from build123d import *

# Parameters (mm, degrees)
F2_W          = 2.032
F2_H          = 3.556
F2_W_2        = 3.556
F2_H_2        = 2.032
F3_DEPTH      = 25.4
F3_DEPTH_BACK = 4.3434


# Not quite as in the source:
# - a feature names something its author has since deleted; it is built from what else it names


with BuildPart() as f1:
    # F0 (on Front) → F1 (revolve)
    with BuildSketch(Plane.XZ):
        with BuildLine():
            ThreePointArc((8.3732076521, 7.5855466623), (7.9877835669, 8.7130510839), (6.9264967271, 9.2547965866))
            Line((6.9264967271, 9.2547965866), (-0.5167923479, 9.906))
            Line((-0.5167923479, 9.906), (-4.3267923479, 9.906))
            Line((-4.3267923479, 9.906), (-4.3267923479, 8.73125))
            Line((-4.3267923479, 8.73125), (-7.5017923479, 8.73125))
            Line((-7.5017923479, 8.73125), (-7.5017923479, 7.5438))
            Line((-7.5017923479, 7.5438), (-13.4549173479, 7.5438))
            ThreePointArc((-13.4549173479, 7.5438), (-13.7355503517, 7.4275580038), (-13.8517923479, 7.146925))
            Line((-13.8517923479, 7.146925), (-13.8517923479, 6.5024))
            Line((-13.8517923479, 6.5024), (8.3732076521, 6.5024))
            Line((8.3732076521, 6.5024), (8.3732076521, 7.5855466623))
        make_face()
    revolve(axis=Axis((-0.2325048039, 0, 0), (1, 0, 0)))

    # F2 (on Right) → F3 (cut, two sides)
    with BuildSketch(Plane.YZ) as f3_sk:
        with Locations((0, -8.1534)):
            Rectangle(F2_W, F2_H)
        with Locations((0, 8.1534)):
            Rectangle(F2_W, F2_H)
        with Locations((-8.1534, 0)):
            Rectangle(F2_W_2, F2_H_2)
        with Locations((8.1534, 0)):
            Rectangle(F2_W_2, F2_H_2)
    extrude(amount=F3_DEPTH, mode=Mode.SUBTRACT)
    extrude(f3_sk.sketch, amount=-F3_DEPTH_BACK, mode=Mode.SUBTRACT)


solid = f1.part
The model under review builds one solid part; all positions refer to its coordinate system, in mm. A direction names the side the tool comes from. Coordinates: 2 decimals unless noted, no trailing zeros. Write each loop counter-clockwise with the first axis right and the second up, starting at its lowest first coordinate (ties: lowest second). Pieces come first, ordered by that corner, then holes. Notation, with made-up numbers: M 54.25,1 L 76.25,1 A21 cw 76.25,29 Z; hole C -29.75,19.25 d3. An arc over 180 degrees is marked long. Put each result on its own line as item: value.
1) Add section D-D on x = -10. Give the boundary of the cut face in (y, z), then the cut area to 3 significant figures.
Computed:
outline: C 0,0 d15.09; hole C 0,0 d13
area: 46.0 mm2
2) For faces 1 (the flat face through (2, 1.016, 8)), 2 (the flat face through (2, -8, 1.016)), 3 (the flat face through (-7.502, 4, -7)), list the 3-axis set-ups (+Z, -Z, +X, -X, +Y, -Y) from which the entire face can be reached by the end or side of a thin tool; tool diameter is ignored.
Computed:
face 1: +Z, -Z, +X
face 2: +X, +Y, -Y
face 3: -X
3) Add section B-B on x = -2.75. Give the boundary of the cut face in (y, z), then the cut area to 3 significant figures.
Computed:
outline: M -9.85,-1.02 A9.91 ccw -1.02,-9.85 L -1.02,-6.42 A6.5 cw -6.42,-1.02 Z; M -9.85,1.02 L -6.42,1.02 A6.5 cw -1.02,6.42 L -1.02,9.85 A9.91 ccw Z; M 1.02,-9.85 A9.91 ccw 9.85,-1.02 L 6.42,-1.02 A6.5 cw 1.02,-6.42 Z; M 1.02,6.42 A6.5 cw 6.42,1.02 L 9.85,1.02 A9.91 ccw 1.02,9.85 Z
area: 148 mm2
4) Clearance check with flat-ended pins moving along their axes: pin 1 Ø4 at (x, z) = (1, -9) entering from -Y; pin 2 Ø1 at (y, z) = (0, -7.5) entering from +X; pin 3 Ø4 at (x, z) = (2, -8.5) entering from +Y; pin 4 Ø4 at (y, z) = (0, 3.5) entering from +X. State where each tip first meets the part, or that it passes through.
Computed:
pin 1: stops at y = -6.84
pin 2: stops at x = -4.34
pin 3: stops at y = 7.2
pin 4: passes through
5) Draft analysis for pull direction Y (two halves, no side actions). For faces 4 (the flat face through (-4.343, 0, -8)), 5 (the cylindrical face through (-2.45, 6.94, -7.07)), 6 (the flat face through (8.373, -5, 5)), state which applies: released by +Y, released by -Y, zero draft, split by the parting line, or undercut.
Computed:
face 4: undercut
face 5: released by +Y
face 6: zero draft
6) Add section A-A on z = 0. Give the boundary of the cut face in (x, y), then the cut area to 3 significant figures.
Computed:
outline: M -13.85,-7.15 A0.4 ccw -13.45,-7.54 L -7.5,-7.54 L -7.5,-8.73 L -4.34,-8.73 L -4.34,-6.5 L -13.85,-6.5 Z; M -13.85,6.5 L -4.34,6.5 L -4.34,8.73 L -7.5,8.73 L -7.5,7.54 L -13.45,7.54 A0.4 ccw -13.85,7.15 Z
area: 27.2 mm2
7) Wall thickness on probe 1 along Y at (x, z) = (-8, 0); probe 2 along Y at (x, z) = (-4.75, 0): over which ranges is each line inside the solid? List them lowest first. Write a range as [from, to].
Computed:
probe 1: y = [-7.54, -6.5], [6.5, 7.54]
probe 2: y = [-8.73, -6.5], [6.5, 8.73]
